Geometry: final body of the model. Coordinates: model frame, mm. Face numbers are marked on the shaded views. A direction names the side the tool comes from. Round coordinates to 2 decimals unless told otherwise and drop trailing zeros. Loops run counter-clockwise (first coordinate to the right, second up) from the corner with the lowest first, then second, coordinate; pieces in that order, holes last. Notation, with made-up numbers: (51, 69.5) - (68, 69.5) arc R12 ccw to (68, 86.5) - close; hole circle Ø1 at (-23.75, 28). An arc over 180 degrees is marked (long way). Return JSON: item names as keys, results as strings. Group by question number.
1. First-contact query: pin 1 Ø9.5 at (y, z) = (-16, 41) entering from -X; pin 2 Ø4 at (x, y) = (10, -29) entering from -Z; pin 3 Ø1.5 at (x, y) = (54.5, -28) entering from +Z. Flat tips, straight axial feed; report the tip coordinate or a pass-through.
2. Section C-C on y = 25. Return loops of the section in (x, z).
3. Section D-D on y = -29. Count the separate pieces of the cut face and the enclosed holes in it, and give its area (3 significant figures).
4. Set-up query: the marked faces 1, 2 and 3. Return all of +Z, -Z, +X, -X, +Y, -Y with unobstructed straight access to the full face (end or side cutting, diameter ignored); none if empty.
5. Section B-B on z = 77. Return loops of the section in (x, y), and give its area (3 significant figures).
6. Material intervals for probe 1 along X at (y, z) = (29, 5.25); probe 2 along Z at (x, y) = (6, -7.5); probe 3 along Z at (x, y) = (40, -3), sorted ascending.
7. Section A-A on x = 55. Return loops of the section in (y, z), and give its area (3 significant figures).
8. Draft query along Z for the marked faces 4, 5 and 6. Return one class per face: +Z half, -Z half, draft (parallel to the pull), parting line (faces both ways), or undercut.
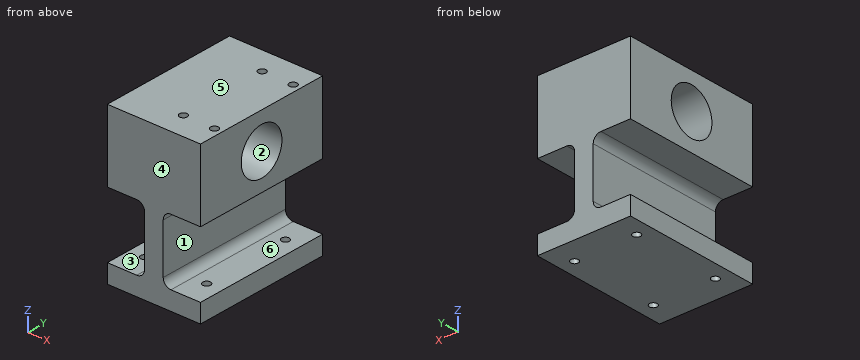
from build123d import *

# Parameters (mm, degrees)
F1_DEPTH      = 45
F1_DEPTH_BACK = 45
F2_R          = 5
F3_R          = 15
F4_DEPTH      = 60
F5_R          = 2.5
F6_DEPTH      = 12
F7_R          = 2.5
F8_DEPTH      = 20


with BuildPart() as f1:
    # F0 (on Front) → F1 (new body, two sides)
    with BuildSketch(Plane.XZ) as f1_sk:
        Polygon((0, 12), (0, 0), (60, 0), (60, 12), (36, 12), (36, 54), (60, 54), (60, 100), (0, 100), (0, 54), (24, 54), (24, 12), align=None)
    extrude(amount=F1_DEPTH)
    extrude(f1_sk.sketch, amount=-F1_DEPTH_BACK)

    # F2
    f2_edges = [f1.edges().sort_by_distance(p)[0] for p in [
        (36, 0, 54),
        (36, 0, 12),
        (24, 0, 12),
        (24, 0, 54),
    ]]
    fillet(f2_edges, radius=F2_R)

    # F3 (on face) → F4 (cut)
    with BuildSketch(Plane.YZ.offset(60)):
        with Locations((0, 77)):
            Circle(F3_R)
    extrude(amount=-F4_DEPTH, mode=Mode.SUBTRACT)

    # F5 (on face) → F6 (cut)
    with BuildSketch(Plane(origin=(0, 0, 0), x_dir=(1, 0, 0), z_dir=(0, 0, -1))):
        with Locations((10, 29)):
            Circle(F5_R)
        with Locations((10, -29)):
            Circle(F5_R)
        with Locations((50, -29)):
            Circle(F5_R)
        with Locations((50, 29)):
            Circle(F5_R)
    extrude(amount=-F6_DEPTH, mode=Mode.SUBTRACT)

    # F7 (on face) → F8 (cut)
    with BuildSketch(Plane.XY.offset(100)):
        with Locations((35, 29)):
            Circle(F7_R)
        with Locations((55, 29)):
            Circle(F7_R)
        with Locations((55, -29)):
            Circle(F7_R)
        with Locations((35, -29)):
            Circle(F7_R)
    extrude(amount=-F8_DEPTH, mode=Mode.SUBTRACT)


solid = f1.part
Taken from the geometry:
{
 "1": {"pin 1": "x = 24", "pin 2": "z = 54", "pin 3": "z = 80"},
 "2": {"outline": "(0, 0) - (60, 0) - (60, 12) - (41, 12) arc R5 cw to (36, 17) - (36, 49) arc R5 cw to (41, 54) - (60, 54) - (60, 100) - (0, 100) - (0, 54) - (19, 54) arc R5 cw to (24, 49) - (24, 17) arc R5 cw to (19, 12) - (0, 12) - close"},
 "3": {"separate pieces": "3", "enclosed holes": "0", "area": "3,690 mm2"},
 "4": {"face 1": "+X, +Y, -Y", "face 2": "+X, -X", "face 3": "-X, +Y, -Y"},
 "5": {"outline": "(0, -45) - (60, -45) - (60, -15) - (0, -15) - close; (0, 15) - (60, 15) - (60, 45) - (0, 45) - close", "area": "3,600 mm2"},
 "6": {"probe 1": "0 to 7.5, 12.5 to 47.5, 52.5 to 60", "probe 2": "0 to 12, 54 to 64.01, 89.99 to 100", "probe 3": "0 to 12.1, 53.9 to 62.3, 91.7 to 100"},
 "7": {"outline": "(-45, 0) - (45, 0) - (45, 12) - (-45, 12) - close; (-45, 54) - (45, 54) - (45, 100) - (31.5, 100) - (31.5, 80) - (26.5, 80) - (26.5, 100) - (-26.5, 100) - (-26.5, 80) - (-31.5, 80) - (-31.5, 100) - (-45, 100) - close; hole circle Ø30 at (0, 77)", "area": "4,310 mm2"},
 "8": {"face 4": "draft", "face 5": "+Z half", "face 6": "undercut"}
}
